Read the model definition and answer for the solid it produces. Units are mm, in the model's axes. Face numbers are marked on the shaded views. A direction names the side the tool comes from. Round coordinates to 2 decimals unless told otherwise and drop trailing zeros. Write each loop counter-clockwise with the first axis right and the second up, starting at its lowest first coordinate (ties: lowest second). Pieces come first, ordered by that corner, then holes.
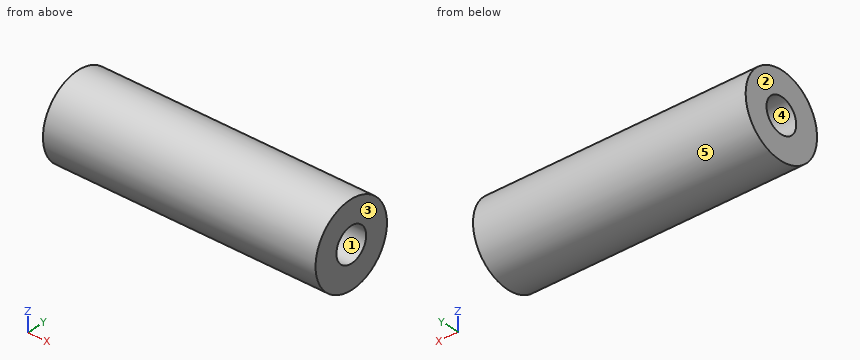
Autodesk Inventor part; units mm, degrees
ref_plane "YZ Plane" through (0, 0, 0) normal (1, 0, 0) x (0, 1, 0)
ref_plane "XZ Plane" through (0, 0, 0) normal (0, 1, 0) x (-1, 0, 0)
ref_plane "XY Plane" through (0, 0, 0) normal (0, 0, 1) x (1, 0, 0)
sketch "Sketch1" plane through (0, 0, 0) normal (1, 0, 0) x (0, 1, 0)
  circle A0 centre (0, 0) radius 4.7625
  dimension "d0" = 9.525
extrude "Extrusion1" add sketch "Sketch1" along normal blind 31.8567
sketch "Sketch2" plane through (31.8567, 0, 0) normal (1, 0, 0) x (0, 0, -1)
  point P0 (0, 0)
  point P1 (0, 0)
hole "Hole1" at (31.8567, 0, 0) direction (-1, 0, 0) diameter 3.9624 depth 13.6144 tip angle 118
sketch "Sketch3" plane through (0, 0, 0) normal (-1, 0, 0) x (0, 0, 1)
  circle A0 centre (0, 0) radius 1.9812
hole "Hole2" at (0, 0, 0) direction (1, 0, 0) diameter 3.9624 depth 13.6144 tip angle 118
properties part number "STOCK,ROUND,0.375inOD,10-32,STANDOFF" material "Aluminum 6061"
Q1. Flat-ended cylindrical pins translate along their axes: pin 1 Ø2 at (x, z) = (12, 1.5) entering from +Y; pin 2 Ø2 at (x, z) = (11.5, -2.5) entering from -Y; pin 3 Ø5 at (x, y) = (11, 3.5) entering from -Z. Find the tip coordinate at first contact, or state that the pin passes through.
Verdict:
pin 1: stops at y = 4.74
pin 2: stops at y = -4.52
pin 3: stops at z = -4.66
Q2. Section D-D (z = -3.25) is taken. Determine the outline of the cut face in (x, y).
Verdict:
outline: (0, -3.48) - (31.86, -3.48) - (31.86, 3.48) - (0, 3.48) - close
Q3. Determine the mould class of the marked faces 3, 4 and 5 for opening direction Z: pulls with the +Z half, pulls with the -Z half, needs draft (parallel to the pull), parting line crosses it, or undercut.
Verdict:
face 3: needs draft
face 4: undercut
face 5: parting line crosses it
Q4. Which of the six approach directions +Z, -Z, +X, -X, +Y, -Y give full straight-line access (tool end or side, diameter ignored) to the marked faces 1 and 2?
Verdict:
face 1: +X
face 2: +Z, -Z, -X, +Y, -Y
Q5. Section B-B (x = 16) is taken. Determine the outline of the cut face in (y, z) (1 decimal).
Verdict:
outline: circle Ø9.5 at (0, 0)
Q6. Section A-A (x = 9.5) is taken. Determine the outline of the cut face in (y, z) (1 decimal), then the cut area to 3 significant figures.
Verdict:
outline: circle Ø9.5 at (0, 0); hole circle Ø4 at (0, 0)
area: 58.9 mm2
Q7. Section C-C (y = 3.5) is taken. Determine the outline of the cut face in (x, z), then the cut area to 3 significant figures.
Verdict:
outline: (0, -3.23) - (31.86, -3.23) - (31.86, 3.23) - (0, 3.23) - close
area: 206 mm2
Q8. Straight lines are drawn through the part: probe 1 along Z at (x, y) = (10.5, 0); probe 2 along Z at (x, y) = (24.5, -1.25); probe 3 along Y at (x, z) = (7, -1). For each, find the intervals that lie inside material, in ascending order.
Verdict:
probe 1: z = -4.76 to -1.98, 1.98 to 4.76
probe 2: z = -4.6 to -1.54, 1.54 to 4.6
probe 3: y = -4.66 to -1.71, 1.71 to 4.66
